```python
from build123d import *

# Parameters (mm, degrees)
SKETCH1_R           = 1.15
BOSS_EXTRUDE1_DEPTH = 5.8
EXTRUDE_THIN1_DEPTH = 5.8


with BuildPart() as part:
    # Sketch1 → Boss-Extrude1 (new body)
    with BuildSketch(Plane.XY):
        Polygon((-6.4, -2.9), (-4.565838245, -2.9), (-4.565838245, -3.592341201), (-1.934161755, -3.592341201), (-1.934161755, -2.9), (1.934161755, -2.9), (1.934161755, -3.592341201), (4.565838245, -3.592341201), (4.565838245, -2.9), (6.4, -2.9), (6.4, 2.9), (-6.4, 2.9), align=None)
        with Locations((-3.25, -2.2)):
            Circle(SKETCH1_R, mode=Mode.SUBTRACT)
        with Locations((3.25, -2.2)):
            Circle(SKETCH1_R, mode=Mode.SUBTRACT)
    extrude(amount=-BOSS_EXTRUDE1_DEPTH)

    # Sketch2 → Extrude-Thin1 (add)
    with BuildSketch(Plane.XY):
        Polygon((-5.4, 2.9), (7.557079146, 6.69), (7.58515322, 6.594021636), (-5.371925926, 2.804021636), align=None)
    extrude(amount=-EXTRUDE_THIN1_DEPTH)


solid = part.part
```
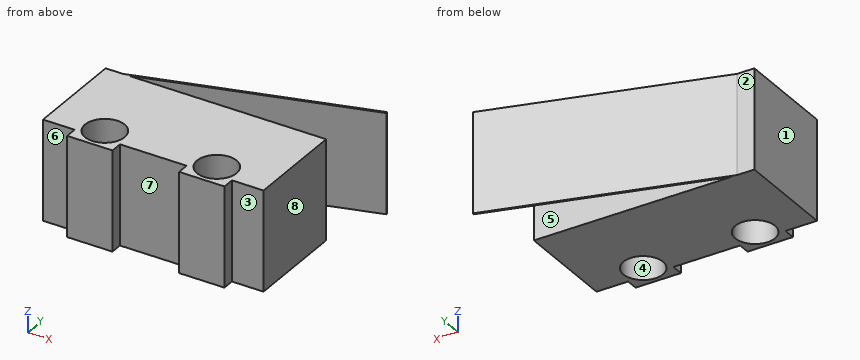
Model file for the job. Use its own axes, mm. Face numbers are marked on the shaded views. A direction names the side the tool comes from. Coordinates: 2 decimals unless noted, no trailing zeros. Write each loop counter-clockwise with the first axis right and the second up, starting at its lowest first coordinate (ties: lowest second). Pieces come first, ordered by that corner, then holes. Notation, with made-up numbers: (-3, -17) - (39, -17) arc R30 cw to (39, 13) - close; hole circle Ø7 at (12.5, 54.5). An arc over 180 degrees is marked (long way). One line per item, written item: value. Start each with the question number.
1. Slice it at C-C (x = 5.5). Write the cut outline in (y, z).
2. Flat gauge pins, fed straight in: pin 1 (0.5 mm diameter, centred on x = -6, z = -3, fed in from +Y); pin 2 (0.6 mm diameter, centred on x = -5, z = -2.5, fed in from -Y); pin 3 (3 mm diameter, centred on y = 0, z = -3, fed in from +X). Where does each tip first touch, or does it go through?
3. Slice it at D-D (x = -3.25). Write the cut outline in (y, z).
4. Mould opens along X. For the marked faces 6, 7 and 8 say: released by +X, released by -X, zero draft, split by the parting line, or undercut.
5. Tool access for the marked faces 1, 2, 3, 4 and 5: list every direction of +Z, -Z, +X, -X, +Y, -Y with a clear straight run to the whole face (end or side of a thin tool).
6. Slice it at B-B (z = -0.4). Write the cut outline in (x, y), plus the area to 3 significant figures.
7. Slice it at A-A (y = -2.2). Write the cut outline in (x, z).
8. Probe line 1 (X direction, y = -3, z = -3.5); line 2 (X direction, y = -1.75, z = -1.05); line 3 (X direction, y = -0.5, z = -4.5). List the from-to ranges inside material, lowest first. Write a range as from..to.
Answers below:
1. outline: (-2.9, -5.8) - (2.9, -5.8) - (2.9, 0) - (-2.9, 0) - close; (5.98, -5.8) - (6.09, -5.8) - (6.09, 0) - (5.98, 0) - close
2. pin 1: stops at y = 2.9
2. pin 2: stops at y = -2.9
2. pin 3: stops at x = 6.4
3. outline: (-3.59, -5.8) - (-3.35, -5.8) - (-3.35, 0) - (-3.59, 0) - close; (-1.05, -5.8) - (2.9, -5.8) - (2.9, 0) - (-1.05, 0) - close; (3.42, -5.8) - (3.53, -5.8) - (3.53, 0) - (3.42, 0) - close
4. face 6: zero draft
4. face 7: undercut
4. face 8: released by +X
5. face 1: +Z, -Z, -X, +Y, -Y
5. face 2: +Z, -Z, -X, +Y
5. face 3: +Z, -Z, +X, -Y
5. face 4: +Z, -Z
5. face 5: +Z, -Z, +X
6. outline: (-6.4, -2.9) - (-4.57, -2.9) - (-4.57, -3.59) - (-1.93, -3.59) - (-1.93, -2.9) - (1.93, -2.9) - (1.93, -3.59) - (4.57, -3.59) - (4.57, -2.9) - (6.4, -2.9) - (6.4, 2.9) - (-5.04, 2.9) - (7.59, 6.59) - (7.56, 6.69) - (-5.4, 2.9) - (-6.4, 2.9) - close; hole circle Ø2.3 at (-3.25, -2.2); hole circle Ø2.3 at (3.25, -2.2)
6. area: 70.9 mm^2
7. outline: (-6.4, -5.8) - (-4.4, -5.8) - (-4.4, 0) - (-6.4, 0) - close; (-2.1, -5.8) - (2.1, -5.8) - (2.1, 0) - (-2.1, 0) - close; (4.4, -5.8) - (6.4, -5.8) - (6.4, 0) - (4.4, 0) - close
8. line 1: x = -4.57..-4.08, -2.42..-1.93, 1.93..2.42, 4.08..4.57
8. line 2: x = -6.4..-4.31, -2.19..2.19, 4.31..6.4
8. line 3: x = -6.4..6.4
